For this review, take the finished solid that the model builds, in its own axes (mm). Coordinates: 2 decimals unless noted, no trailing zeros. Answer as a JSON object with one key per item and string values. Group by question number.
1) For pin 1 (0.6 mm diameter, centred on x = -9.5, z = 136, fed in from +Y); pin 2 (2 mm diameter, centred on y = 1, z = 112, fed in from -X); pin 3 (0.8 mm diameter, centred on x = -9, z = 113.5, fed in from +Y), all flat-tipped, find the tip position at first contact; note any pin that passes through.
2) Add section A-A, the plane z = 93.5. Count the separate pieces of the cut face and the enclosed holes in it, then the cut area to 3 significant figures.
3) Wall thickness on L1, parallel to X at y = 2, z = 37.5; L2, parallel to X at y = -2.25, z = 111.5; L3, parallel to Y at x = -7.25, z = 174: over which ranges is each line inside the solid? List them lowest first.
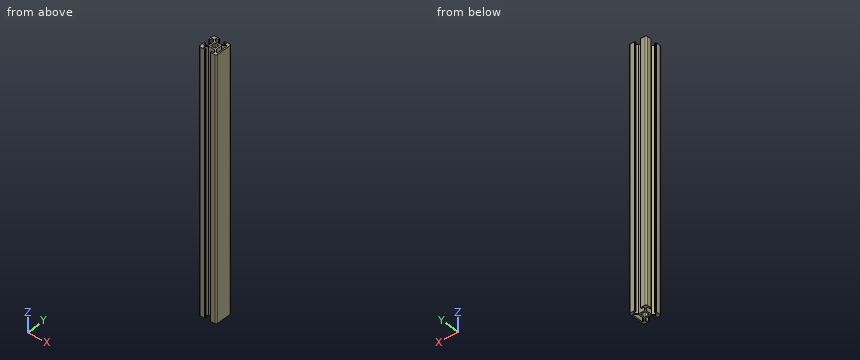
from build123d import *

# Parameters (mm, degrees)
BOSS_EXTRUDE1_DEPTH = 3000
CUT_EXTRUDE1_DEPTH  = 2700


with BuildPart() as part:
    # Sketch1 → Boss-Extrude1 (new body)
    with BuildSketch(Plane.XY):
        with BuildLine():
            Line((-3.43933983, -4.5), (3.43933983, -4.5))
            Line((3.43933983, -4.5), (6, -7.06066017))
            Line((6, -7.06066017), (6, -8.5))
            Line((6, -8.5), (3, -8.5))
            Line((3, -8.5), (3, -9.5))
            Line((3, -9.5), (3.5, -9.5))
            Line((3.5, -9.5), (3.5, -10))
            Line((3.5, -10), (8.5, -10))
            ThreePointArc((8.5, -10), (9.56066017, -9.56066017), (10, -8.5))
            Line((10, -8.5), (10, 8.5))
            ThreePointArc((10, 8.5), (9.56066017, 9.56066017), (8.5, 10))
            Line((8.5, 10), (3.5, 10))
            Line((3.5, 10), (3.5, 9.5))
            Line((3.5, 9.5), (3, 9.5))
            Line((3, 9.5), (3, 8.5))
            Line((3, 8.5), (6, 8.5))
            Line((6, 8.5), (6, 7.06066017))
            Line((6, 7.06066017), (3.43933983, 4.5))
            Line((3.43933983, 4.5), (-3.43933983, 4.5))
            Line((-3.43933983, 4.5), (-6, 7.06066017))
            Line((-6, 7.06066017), (-6, 8.5))
            Line((-6, 8.5), (-3, 8.5))
            Line((-3, 8.5), (-3, 9.5))
            Line((-3, 9.5), (-3.5, 9.5))
            Line((-3.5, 9.5), (-3.5, 10))
            Line((-3.5, 10), (-8.5, 10))
            ThreePointArc((-8.5, 10), (-9.56066017, 9.56066017), (-10, 8.5))
            Line((-10, 8.5), (-10, 3.5))
            Line((-10, 3.5), (-9.5, 3.5))
            Line((-9.5, 3.5), (-9.5, 3))
            Line((-9.5, 3), (-8.5, 3))
            Line((-8.5, 3), (-8.5, 6))
            Line((-8.5, 6), (-7.06066017, 6))
            Line((-7.06066017, 6), (-4.5, 3.43933983))
            Line((-4.5, 3.43933983), (-4.5, -3.43933983))
            Line((-4.5, -3.43933983), (-7.06066017, -6))
            Line((-7.06066017, -6), (-8.5, -6))
            Line((-8.5, -6), (-8.5, -3))
            Line((-8.5, -3), (-9.5, -3))
            Line((-9.5, -3), (-9.5, -3.5))
            Line((-9.5, -3.5), (-10, -3.5))
            Line((-10, -3.5), (-10, -8.5))
            ThreePointArc((-10, -8.5), (-9.56066017, -9.56066017), (-8.5, -10))
            Line((-8.5, -10), (-3.5, -10))
            Line((-3.5, -10), (-3.5, -9.5))
            Line((-3.5, -9.5), (-3, -9.5))
            Line((-3, -9.5), (-3, -8.5))
            Line((-3, -8.5), (-6, -8.5))
            Line((-6, -8.5), (-6, -7.06066017))
            Line((-6, -7.06066017), (-3.43933983, -4.5))
        make_face()
        Polygon((8.5, 6.73223305), (7.79289322, 6.73223305), (4.5, 3.43933983), (4.5, -3.43933983), (7.79289322, -6.73223305), (8.5, -6.73223305), align=None, mode=Mode.SUBTRACT)
        with BuildLine():
            Line((-3.0001742, 1.94957327), (-2.43563636, 1.27678327))
            ThreePointArc((-2.43563636, 1.27678327), (-2.75, 0), (-2.43563636, -1.27678327))
            Line((-2.43563636, -1.27678327), (-3.0001742, -1.94957327))
            Line((-3.0001742, -1.94957327), (-1.94957327, -3.0001742))
            Line((-1.94957327, -3.0001742), (-1.27678327, -2.43563636))
            ThreePointArc((-1.27678327, -2.43563636), (0, -2.75), (1.27678327, -2.43563636))
            Line((1.27678327, -2.43563636), (1.94957327, -3.0001742))
            Line((1.94957327, -3.0001742), (3.0001742, -1.94957327))
            Line((3.0001742, -1.94957327), (2.43563636, -1.27678327))
            ThreePointArc((2.43563636, -1.27678327), (2.75, 0), (2.43563636, 1.27678327))
            Line((2.43563636, 1.27678327), (3.0001742, 1.94957327))
            Line((3.0001742, 1.94957327), (1.94957327, 3.0001742))
            Line((1.94957327, 3.0001742), (1.27678327, 2.43563636))
            ThreePointArc((1.27678327, 2.43563636), (0, 2.75), (-1.27678327, 2.43563636))
            Line((-1.27678327, 2.43563636), (-1.94957327, 3.0001742))
            Line((-1.94957327, 3.0001742), (-3.0001742, 1.94957327))
        make_face(mode=Mode.SUBTRACT)
    extrude(amount=BOSS_EXTRUDE1_DEPTH)

    # Sketch2 → Cut-Extrude1 (cut)
    with BuildSketch(Plane.XY.offset(3000)):
        with BuildLine():
            Line((-6, -7.06066017), (-3.43933983, -4.5))
            Line((-3.43933983, -4.5), (3.43933983, -4.5))
            Line((3.43933983, -4.5), (6, -7.06066017))
            Line((6, -7.06066017), (6, -8.5))
            Line((6, -8.5), (3, -8.5))
            Line((3, -8.5), (3, -9.5))
            Line((3, -9.5), (3.5, -9.5))
            Line((3.5, -9.5), (3.5, -10))
            Line((3.5, -10), (8.5, -10))
            ThreePointArc((8.5, -10), (9.56066017, -9.56066017), (10, -8.5))
            Line((10, -8.5), (10, 8.5))
            ThreePointArc((10, 8.5), (9.56066017, 9.56066017), (8.5, 10))
            Line((8.5, 10), (3.5, 10))
            Line((3.5, 10), (3.5, 9.5))
            Line((3.5, 9.5), (3, 9.5))
            Line((3, 9.5), (3, 8.5))
            Line((3, 8.5), (6, 8.5))
            Line((6, 8.5), (6, 7.06066017))
            Line((6, 7.06066017), (3.43933983, 4.5))
            Line((3.43933983, 4.5), (-3.43933983, 4.5))
            Line((-3.43933983, 4.5), (-6, 7.06066017))
            Line((-6, 7.06066017), (-6, 8.5))
            Line((-6, 8.5), (-3, 8.5))
            Line((-3, 8.5), (-3, 9.5))
            Line((-3, 9.5), (-3.5, 9.5))
            Line((-3.5, 9.5), (-3.5, 10))
            Line((-3.5, 10), (-8.5, 10))
            ThreePointArc((-8.5, 10), (-9.56066017, 9.56066017), (-10, 8.5))
            Line((-10, 8.5), (-10, 3.5))
            Line((-10, 3.5), (-9.5, 3.5))
            Line((-9.5, 3.5), (-9.5, 3))
            Line((-9.5, 3), (-8.5, 3))
            Line((-8.5, 3), (-8.5, 6))
            Line((-8.5, 6), (-7.06066017, 6))
            Line((-7.06066017, 6), (-4.5, 3.43933983))
            Line((-4.5, 3.43933983), (-4.5, -3.43933983))
            Line((-4.5, -3.43933983), (-7.06066017, -6))
            Line((-7.06066017, -6), (-8.5, -6))
            Line((-8.5, -6), (-8.5, -3))
            Line((-8.5, -3), (-9.5, -3))
            Line((-9.5, -3), (-9.5, -3.5))
            Line((-9.5, -3.5), (-10, -3.5))
            Line((-10, -3.5), (-10, -8.5))
            ThreePointArc((-10, -8.5), (-9.56066017, -9.56066017), (-8.5, -10))
            Line((-8.5, -10), (-3.5, -10))
            Line((-3.5, -10), (-3.5, -9.5))
            Line((-3.5, -9.5), (-3, -9.5))
            Line((-3, -9.5), (-3, -8.5))
            Line((-3, -8.5), (-6, -8.5))
            Line((-6, -8.5), (-6, -7.06066017))
        make_face()
    extrude(amount=-CUT_EXTRUDE1_DEPTH, mode=Mode.SUBTRACT)


solid = part.part
Output values:
{
 "1": {"pin 1": "stops at y = 9.83", "pin 2": "stops at x = -4.5", "pin 3": "stops at y = 10"},
 "2": {"separate pieces": "1", "enclosed holes": "2", "area": "174 mm²"},
 "3": {"L1": "x = -4.5 to -2.95, 2.95 to 4.5, 8.5 to 10", "L2": "x = -4.5 to -2.7, 2.7 to 4.5, 8.5 to 10", "L3": "y = -10 to -6, 6 to 10"}
}
